For this review, take the finished solid that the model builds, in its own axes (mm). Face numbers are marked on the shaded views. Give positions to 0.01 mm unless a question says otherwise; leave off trailing zeros. Write each loop counter-clockwise with the first axis right and the second up, starting at its lowest first coordinate (ties: lowest second). Pieces come first, ordered by that corner, then holes. Notation, with made-up numbers: (41, 35.25) -> (82, 35.25) arc R15 ccw to (82, 60.25) -> close; hole circle Ø5 at (23, 70). An arc over 180 degrees is marked (long way). Return JSON: item names as keys, results as strings.
from build123d import *

# Parameters (mm, degrees)
SKETCH_1_W          = 19
SKETCH_1_H          = 19
SKETCH_1_W_2        = 15.88
SKETCH_1_H_2        = 15.88
EXTRUDE_1_DEPTH     = 900
FILLET_2_R          = 1
SKETCH_2_W          = 650
SKETCH_2_H          = 19
CUT_EXTRUDE_2_DEPTH = 51


with BuildPart() as part:
    # 스케치1 → 보스-돌출1 (new body)
    with BuildSketch(Plane.XY):
        with Locations((9.5, -9.5)):
            Rectangle(SKETCH_1_W, SKETCH_1_H)
        with Locations((9.5, -9.5)):
            Rectangle(SKETCH_1_W_2, SKETCH_1_H_2, mode=Mode.SUBTRACT)
    extrude(amount=EXTRUDE_1_DEPTH)

    # 필렛2
    fillet_2_edges = [part.edges().sort_by_distance(p)[0] for p in [
        (0, 0, 450),
        (19, 0, 450),
        (19, -19, 450),
        (0, -19, 450),
    ]]
    fillet(fillet_2_edges, radius=FILLET_2_R)

    # 스케치2 → 컷-돌출2 (cut)
    with BuildSketch(Plane(origin=(19, 0, 0), x_dir=(0, 0, -1), z_dir=(1, 0, 0))):
        with Locations((-575, -9.5)):
            Rectangle(SKETCH_2_W, SKETCH_2_H)
    extrude(amount=-CUT_EXTRUDE_2_DEPTH, mode=Mode.SUBTRACT)


solid = part.part
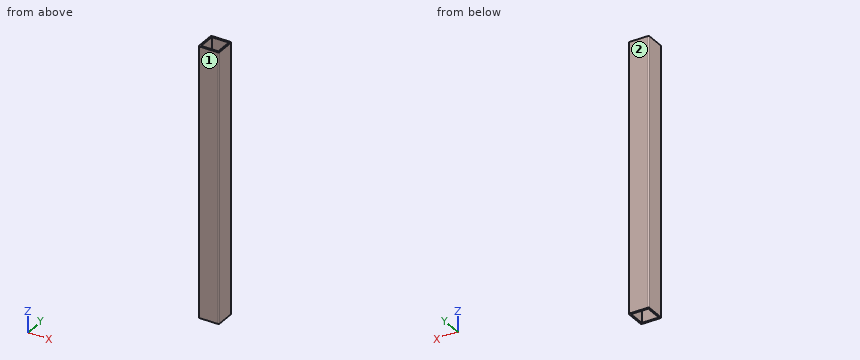
1. Add section C-C, the plane z = 213. State the section outline as (x, y) points, plus the area to 3 significant figures.
Results found:
{"outline": "(0, -18) arc R1 ccw to (1, -19) -> (18, -19) arc R1 ccw to (19, -18) -> (19, -1) arc R1 ccw to (18, 0) -> (1, 0) arc R1 ccw to (0, -1) -> close; hole (1.56, -17.44) -> (17.44, -17.44) -> (17.44, -1.56) -> (1.56, -1.56) -> close", "area": "108 mm²"}
2. For pin 1 (3 mm diameter, centred on x = 17, y = -4.5, fed in from -Z), flat-tipped, find the tip position at first contact; note if it passes through.
Results found:
{"pin 1": "stops at z = 0"}
3. Add section A-A, the plane y = -13.75. State the section outline as (x, z) points, plus the area to 3 significant figures.
Results found:
{"outline": "(0, 0) -> (1.56, 0) -> (1.56, 250) -> (0, 250) -> close; (17.44, 0) -> (19, 0) -> (19, 250) -> (17.44, 250) -> close", "area": "780 mm²"}
4. Add section B-B, the plane x = 4. State the section outline as (y, z) points.
Results found:
{"outline": "(-19, 0) -> (-17.44, 0) -> (-17.44, 250) -> (-19, 250) -> close; (-1.56, 0) -> (0, 0) -> (0, 250) -> (-1.56, 250) -> close"}
5. To check wall thickness, follow probe 1 along Y at (x, z) = (15.5, 62); probe 2 along X at (y, z) = (-6.25, 207); probe 3 along Y at (x, z) = (18.25, 46.5). State the ranges of each line that lie inside material, in increasing order.
Results found:
{"probe 1": "y = -19 to -17.44, -1.56 to 0", "probe 2": "x = 0 to 1.56, 17.44 to 19", "probe 3": "y = -18.97 to -0.03"}
6. The part is to be moulded in two halves that separate along Y. For the marked faces 1 and 2, say which applies: +Y half, -Y half, draft (parallel to the pull), parting line (faces both ways), or undercut.
Results found:
{"face 1": "-Y half", "face 2": "+Y half"}
